Could you check a few things on this model? Use its own coordinates, in mm. Face numbers are marked on the shaded views. A direction names the side the tool comes from. Give positions to 0.01 mm unless a question says otherwise; leave off trailing zeros. Loops run counter-clockwise (first coordinate to the right, second up) from the corner with the lowest first, then second, coordinate; pieces in that order, holes last. Notation, with made-up numbers: (44, 29.25) - (81, 29.25) arc R31 ccw to (81, 65.25) - close; hole circle Ø1 at (-7, 56.25). An arc over 180 degrees is marked (long way). Write each question's results on one line, items separated by ' | '. Start each with the question number.
(1) Suppose I cut it at A-A (y = -28.5). Please give me the cut outline in (x, z).
(2) On a 3-axis mill with a long thin cutter (end or side, diameter ignored), from which of +Z, -Z, +X, -X, +Y, -Y can I reach the whole of each face in a straight line? I mean the marked faces 1, 2, 3 and 4. Say none if no direction works.
(3) I need wall thicknesses on line 1 (Z direction, x = 0, y = -3); line 2 (X direction, y = -20, z = 25); line 3 (Y direction, x = -15, z = 29). Which ranges of each line are inside material? Lowest first, please.
(4) For pin 1 (3 mm diameter, centred on x = -32.5, y = -4, fed in from -Z); pin 2 (2 mm diameter, centred on x = 2, z = 4, fed in from -Y); pin 3 (3 mm diameter, centred on x = 14, y = -23.5, fed in from -Z); pin 4 (3 mm diameter, centred on x = -15.5, y = -13, fed in from -Z), each with a flat end and sliding along its axis, tell me the tip position at first contact or that it passes through.
(5) Suppose I cut it at C-C (x = 4). Please give me the cut outline in (y, z).
(6) Suppose I cut it at D-D (x = -26.5). Please give me the cut outline in (y, z), and give its area (3 significant figures).
(7) If we mould it in two halves opening along X, with no side actions, what happens to the marked faces 5, 6 and 7? For each: released by +X, released by -X, zero draft, split by the parting line, or undercut.
(8) Suppose I cut it at B-B (x = 15.5). Please give me the cut outline in (y, z).
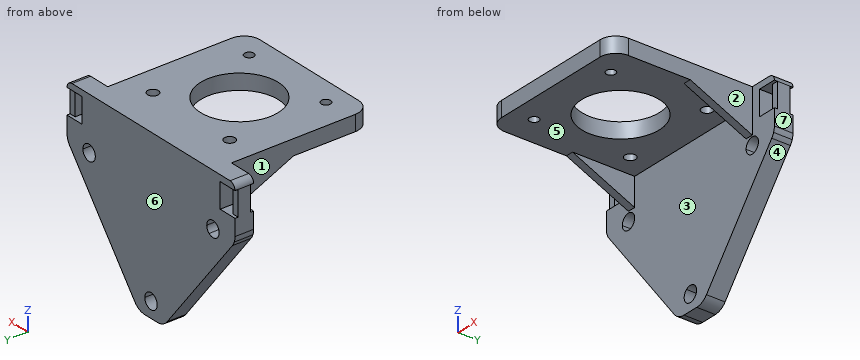
from build123d import *

# Parameters (mm, degrees)
F0_W      = 4
F0_H      = 8
F0_W_2    = 2
F1_DEPTH  = 6
F2_W      = 2
F2_H      = 8
F3_DEPTH  = 1
F4_W      = 2
F4_H      = 8
F5_DEPTH  = 1
F6_W      = 25
F6_H      = 5
F7_DEPTH  = 45
F8_R      = 5.08
F9_W      = 2.5
F9_H      = 20
F10_DEPTH = 9
F12_DEPTH = 50.292
F13_R     = 12.5
F13_R_2   = 1.75
F13_R_3   = 1.5
F14_DEPTH = 25.4


# Not quite as in the source:
# - a feature names something its author has since deleted; it is built from what else it names


with BuildPart() as f1:
    # F0 (on Front) → F1 (new body)
    with BuildSketch(Plane.XZ):
        with BuildLine():
            Line((-22.5, 15.1779663801), (-15.95, 15.1779663801))
            Line((-15.95, 15.1779663801), (15.95, 15.1779663801))
            Line((15.95, 15.1779663801), (22.5, 15.1779663801))
            ThreePointArc((22.5, 15.1779663801), (25, 17.6779663801), (27.5, 15.1779663801))
            Line((27.5, 15.1779663801), (33.6112053721, 15.1779663801))
            ThreePointArc((33.6112053721, 15.1779663801), (33.8410734014, 16.027307097), (33.9184952978, 16.9037914461))
            Line((33.9184952978, 16.9037914461), (33.9184952978, 19.2973875134))
            Line((33.9184952978, 19.2973875134), (33.9184952978, 20.1779663801))
            Line((33.9184952978, 20.1779663801), (33.0379164311, 20.1779663801))
            Line((33.0379164311, 20.1779663801), (-32.6408470514, 20.1779663801))
            Line((-32.6408470514, 20.1779663801), (-33.9184952978, 20.1779663801))
            Line((-33.9184952978, 20.1779663801), (-33.9184952978, 18.9003181337))
            Line((-33.9184952978, 18.9003181337), (-33.9184952978, 16.9037914461))
            ThreePointArc((-33.9184952978, 16.9037914461), (-33.8410734014, 16.027307097), (-33.6112053721, 15.1779663801))
            Line((-33.6112053721, 15.1779663801), (-27.5, 15.1779663801))
            ThreePointArc((-27.5, 15.1779663801), (-25, 17.6779663801), (-22.5, 15.1779663801))
        make_face()
        with BuildLine():
            Line((15.95, 15.1779663801), (-15.95, 15.1779663801))
            Line((-15.95, 15.1779663801), (-22.5, 15.1779663801))
            ThreePointArc((-22.5, 15.1779663801), (-22.7521952698, 14.0837205691), (-23.457899116, 13.2102456521))
            Line((-23.457899116, 13.2102456521), (-1.542100884, -14.7543128919))
            ThreePointArc((-1.542100884, -14.7543128919), (0, -14.2220336199), (1.542100884, -14.7543128919))
            Line((1.542100884, -14.7543128919), (23.457899116, 13.2102456521))
            ThreePointArc((23.457899116, 13.2102456521), (22.7521952698, 14.0837205691), (22.5, 15.1779663801))
            Line((22.5, 15.1779663801), (15.95, 15.1779663801))
        make_face()
        with BuildLine():
            ThreePointArc((-23.457899116, 13.2102456521), (-26.094245811, 12.9301616499), (-27.5, 15.1779663801))
            Line((-27.5, 15.1779663801), (-33.6112053721, 15.1779663801))
            ThreePointArc((-33.6112053721, 15.1779663801), (-33.28570797, 14.4691552359), (-32.8539367538, 13.819589678))
            Line((-32.8539367538, 13.819589678), (-6.5014092727, -19.8062353879))
            ThreePointArc((-6.5014092727, -19.8062353879), (-4.7544594387, -21.2176430802), (-2.5659678166, -21.7220336199))
            Line((-2.5659678166, -21.7220336199), (0, -21.7220336199))
            Line((0, -21.7220336199), (0, -19.2220336199))
            ThreePointArc((0, -19.2220336199), (-2.3631866008, -17.5377229541), (-1.542100884, -14.7543128919))
            Line((-1.542100884, -14.7543128919), (-23.457899116, 13.2102456521))
        make_face()
        with BuildLine():
            Line((33.6112053721, 15.1779663801), (27.5, 15.1779663801))
            ThreePointArc((27.5, 15.1779663801), (26.094245811, 12.9301616499), (23.457899116, 13.2102456521))
            Line((23.457899116, 13.2102456521), (1.542100884, -14.7543128919))
            ThreePointArc((1.542100884, -14.7543128919), (2.2478047302, -15.6277878088), (2.5, -16.7220336199))
            ThreePointArc((2.5, -16.7220336199), (1.767766953, -18.4898005728), (0, -19.2220336199))
            Line((0, -19.2220336199), (0, -21.7220336199))
            Line((0, -21.7220336199), (2.5659678166, -21.7220336199))
            ThreePointArc((2.5659678166, -21.7220336199), (4.7544594387, -21.2176430802), (6.5014092727, -19.8062353879))
            Line((6.5014092727, -19.8062353879), (32.8539367538, 13.819589678))
            ThreePointArc((32.8539367538, 13.819589678), (33.28570797, 14.4691552359), (33.6112053721, 15.1779663801))
        make_face()
        with BuildLine():
            Line((-33.9184952978, 30.1779663801), (-33.9184952978, 20.1779663801))
            Line((-33.9184952978, 20.1779663801), (-32.6408470514, 20.1779663801))
            Line((-32.6408470514, 20.1779663801), (33.0379164311, 20.1779663801))
            Line((33.0379164311, 20.1779663801), (33.9184952978, 20.1779663801))
            Line((33.9184952978, 20.1779663801), (33.9184952978, 22.1779663801))
            Line((33.9184952978, 22.1779663801), (31.9184952978, 22.1779663801))
            Line((31.9184952978, 22.1779663801), (27.9184952978, 22.1779663801))
            Line((27.9184952978, 22.1779663801), (27.9184952978, 30.1779663801))
            Line((27.9184952978, 30.1779663801), (31.9184952978, 30.1779663801))
            Line((31.9184952978, 30.1779663801), (33.9184952978, 30.1779663801))
            ThreePointArc((33.9184952978, 30.1779663801), (33.3327088602, 31.5921799425), (31.9184952978, 32.1779663801))
            Line((31.9184952978, 32.1779663801), (-31.9184952978, 32.1779663801))
            ThreePointArc((-31.9184952978, 32.1779663801), (-33.3327088602, 31.5921799425), (-33.9184952978, 30.1779663801))
        make_face()
        with Locations((-29.9184952978, 26.1779663801)):
            Rectangle(F0_W, F0_H, mode=Mode.SUBTRACT)
        with Locations((32.9184952978, 26.1779663801)):
            Rectangle(F0_W_2, F0_H)
    extrude(amount=F1_DEPTH)

    # F2 (on face) → F3 (cut)
    with BuildSketch(Plane(origin=(0, 0, 0), x_dir=(-1, 0, 0), z_dir=(0, 1, 0))):
        with Locations((-32.9184952978, 26.1779663801)):
            Rectangle(F2_W, F2_H)
        with Locations((32.9184952978, 26.1779663801)):
            Rectangle(F2_W, F2_H)
    extrude(amount=-F3_DEPTH, mode=Mode.SUBTRACT)

    # F4 (on face) → F5 (cut)
    with BuildSketch(Plane.XZ.offset(6)):
        with Locations((-32.9184952978, 26.1779663801)):
            Rectangle(F4_W, F4_H)
        with Locations((32.9184952978, 26.1779663801)):
            Rectangle(F4_W, F4_H)
    extrude(amount=-F5_DEPTH, mode=Mode.SUBTRACT)

    # F6 (on face) → F7 (join)
    with BuildSketch(Plane.XZ.offset(6)):
        with Locations((-12.5, 29.6779663801)):
            Rectangle(F6_W, F6_H)
        with Locations((12.5, 29.6779663801)):
            Rectangle(F6_W, F6_H)
    extrude(amount=F7_DEPTH)

    # F8
    f8_edges = [f1.edges().sort_by_distance(p)[0] for p in [
        (25, -51, 29.677966),
        (-25, -51, 29.677966),
    ]]
    fillet(f8_edges, radius=F8_R)

    # F9 (on face) → F10 (join)
    with BuildSketch(Plane(origin=(0, 0, 27.1779663801), x_dir=(1, 0, 0), z_dir=(0, 0, -1))):
        with Locations((23.75, 16)):
            Rectangle(F9_W, F9_H)
        with Locations((-23.75, 16)):
            Rectangle(F9_W, F9_H)
    extrude(amount=F10_DEPTH)

    # F11 (on face) → F12 (cut)
    with BuildSketch(Plane(origin=(-25, 0, 0), x_dir=(0, -1, 0), z_dir=(-1, 0, 0))):
        Polygon((26, 27.1779663801), (6, 18.1779663801), (26, 18.1779663801), align=None)
    extrude(amount=-F12_DEPTH, mode=Mode.SUBTRACT)

    # F13 (on face) → F14 (cut)
    with BuildSketch(Plane.XY.offset(32.1779663801)):
        with Locations((0, -28.5)):
            Circle(F13_R)
        with Locations((-15.5, -13)):
            Circle(F13_R_2)
        with Locations((15.5, -13)):
            Circle(F13_R_2)
        with Locations((15.5, -44)):
            Circle(F13_R_3)
        with Locations((-15.5, -44)):
            Circle(F13_R_3)
    extrude(amount=-F14_DEPTH, mode=Mode.SUBTRACT)


solid = f1.part
Output values:
1) outline: (-25, 27.18) - (-12.5, 27.18) - (-12.5, 32.18) - (-25, 32.18) - close; (12.5, 27.18) - (25, 27.18) - (25, 32.18) - (12.5, 32.18) - close
2) face 1: +Z, -Z, -X, -Y | face 2: +Z, -Z, +X, -Y | face 3: -Z, -Y | face 4: -Z, +X, +Y, -Y
3) line 1: -21.72 to -19.22, -14.22 to 32.18 | line 2: -25 to -22.5, 22.5 to 25 | line 3: -51 to -45.41, -42.59 to -14.68, -11.32 to 0
4) pin 1: z = 11.45 | pin 2: y = -6 | pin 3: z = 27.18 | pin 4: through
5) outline: (-51, 27.18) - (-40.34, 27.18) - (-40.34, 32.18) - (-51, 32.18) - close; (-16.66, 27.18) - (-6, 27.18) - (-6, -21.51) - (0, -21.51) - (0, 32.18) - (-16.66, 32.18) - close
6) outline: (-6, 5.71) - (0, 5.71) - (0, 13.18) - (-6, 13.18) - close; (-6, 17.18) - (0, 17.18) - (0, 32.18) - (-6, 32.18) - close | area: 135 mm2
7) face 5: undercut | face 6: zero draft | face 7: released by +X
8) outline: (-51, 27.18) - (-45.5, 27.18) - (-45.5, 32.18) - (-51, 32.18) - close; (-42.5, 27.18) - (-14.75, 27.18) - (-14.75, 32.18) - (-42.5, 32.18) - close; (-11.25, 27.18) - (-6, 27.18) - (-6, -8.32) - (0, -8.32) - (0, 32.18) - (-11.25, 32.18) - close
